Build history of the part. All positions in model axes, mm. A direction names the side the tool comes from. Give positions to 0.01 mm unless a question says otherwise; leave off trailing zeros. Write each loop counter-clockwise with the first axis right and the second up, starting at its lowest first coordinate (ties: lowest second). Pieces come first, ordered by that corner, then holes. Notation, with made-up numbers: (12, -27.75) -> (52, -27.75) arc R16 cw to (52, -10.75) -> close; hole circle Ø3 at (-32, 10). An arc over 180 degrees is marked (long way). Write item = value, one per line. Start each with the question number.
Q1. Wall check: line 1 (Y direction, x = 8.5, z = -23); line 2 (Z direction, x = 0, y = -187.5); line 3 (Y direction, x = 20.9, z = 0). Give the ranges that are in metal, low to high.
Q2. Drop flat-ended pins along their axis: P1, Ø1.5, axis at y = -106.5, z = 6.5, coming from the +X side; P2, Ø10, axis at x = -18.5, z = 10.5, coming from the +Y side; P3, Ø10, axis at y = -237, z = 8, coming from the -X side. Give the stop position or say it passes through.
Q3. Saw through at A-A, the plane y = -20. List the corners of the cut face in (x, z), then the cut area to 3 significant figures.
Q4. Tool access for faces 5 (the face through (-9.4, -351, 22.3)), 6 (the face through (-7.956, -414.86, -11.236)), 7 (the face through (22, -124, 0)), 8 (the face through (13.041, -414.86, 4.414)): list every direction of +Z, -Z, +X, -X, +Y, -Y with a clear straight run to the whole face (end or side of a thin tool).
Q5. Saw through at B-B, the plane y = -112. List the corners of the cut face in (x, z).
Q6. Mould opens along Y. For faces 1 (the face through (3, -425, -1)), 2 (the face through (4, -400, 0)), 3 (the face through (5.4, 1.1, 10)), 4 (the face through (23.846, -299.3, 7.509)) say: pulls with the +Y half, pulls with the -Y half, needs draft (parallel to the pull), parting line crosses it, or undercut.
from build123d import *

# Parameters (mm, degrees)
F0_R          = 25
F0_R_2        = 20
F1_DEPTH      = 400
F2_R          = 25
F3_DEPTH      = 5
F5_DEPTH      = 20
F7_D          = 5
F10_D         = 12
F10_DEPTH     = 6
F10_START     = 0.7306779
F10_TIP       = 3.6051637142
F12_DEPTH     = 2
F17_D         = 12
F17_DEPTH     = 6
F17_START     = 0.7306779
F17_TIP       = 3.6051637142
F19_D         = 12
F19_DEPTH     = 6
F19_START     = 0.7306779
F19_TIP       = 3.6051637142
F21_R         = 25
F21_R_2       = 24
F22_DEPTH     = 1
F24_R         = 25
F24_R_2       = 24
F25_DEPTH     = 1
F27_DEPTH     = 20
F28_T1_DEPTH  = 16.0381401647
F28_T3_DEPTH  = 31.2249898061
F28_T5_DEPTH  = 16.0381402184
F28_T7_DEPTH  = 16.0381401647
F28_T9_DEPTH  = 31.2249898061
F28_T11_DEPTH = 16.0381402184
F28_T13_DEPTH = 16.0381401647
F28_T15_DEPTH = 31.2249898061
F28_T17_DEPTH = 16.0381402184


# Not quite as in the source:
# - a fillet or chamfer that OpenCascade refuses, or shapes differently, is made with other operations: its cross-section is extruded or revolved along the edge and cut away or added


with BuildPart() as f1:
    # F0 (on Front) → F1 (new body)
    with BuildSketch(Plane.XZ):
        Circle(F0_R)
        Circle(F0_R_2, mode=Mode.SUBTRACT)
    extrude(amount=F1_DEPTH)

    # F2 (on face) → F3 (join)
    with BuildSketch(Plane.XZ.offset(400)):
        Circle(F2_R)
    extrude(amount=F3_DEPTH)

    # F4 (on face) → F5 (join)
    with BuildSketch(Plane.XZ.offset(405)):
        Polygon((-16.0628025015, -5.6190539991), (0.380358971, -17.013016167), (16.2978772735, -4.8955682433), (9.6922831285, 13.9873885984), (-10.3077168715, 13.540249811), align=None)
    extrude(amount=F5_DEPTH)

    # F7 (through all)
    with Locations(Plane.XZ.offset(425)):
        with Locations((0, 0)):
            Hole(F7_D / 2)

    # F10
    # its depths count from where the whole tool has entered the part; down to there all is cleared
    with Locations(Plane.YZ.offset(25).offset(-F10_START)):
        with Locations((-20, 0), (-130, 0)):
            Hole(F10_D / 2, depth=F10_DEPTH)
            with Locations((0, 0, -(F10_DEPTH + F10_TIP / 2))):  # 118° drill point
                Cone(0, F10_D / 2, F10_TIP, mode=Mode.SUBTRACT)

    # F11 (on face) → F12 (join)
    with BuildSketch(Plane(origin=(0, 0, 0), x_dir=(-1, 0, 0), z_dir=(0, 1, 0))):
        Polygon((12.5, -21.6506350946), (12.5, 21.6506350946), (-25, 0), align=None)
    extrude(amount=F12_DEPTH)

    # F17
    # its depths count from where the whole tool has entered the part; down to there all is cleared
    with Locations(Plane(origin=(-12.5, 0, -21.6506350946), x_dir=(0.8660254038, 0, -0.5), z_dir=(-0.5, 0, -0.8660254038)).offset(-F17_START)):
        with Locations((0, 20), (0, 130)):
            Hole(F17_D / 2, depth=F17_DEPTH)
            with Locations((0, 0, -(F17_DEPTH + F17_TIP / 2))):  # 118° drill point
                Cone(0, F17_D / 2, F17_TIP, mode=Mode.SUBTRACT)

    # F19
    # its depths count from where the whole tool has entered the part; down to there all is cleared
    with Locations(Plane(origin=(-12.5, 0, 21.6506350946), x_dir=(0.8660254038, 0, 0.5), z_dir=(-0.5, 0, 0.8660254038)).offset(-F19_START)):
        with Locations((0, -20), (0, -130)):
            Hole(F19_D / 2, depth=F19_DEPTH)
            with Locations((0, 0, -(F19_DEPTH + F19_TIP / 2))):  # 118° drill point
                Cone(0, F19_D / 2, F19_TIP, mode=Mode.SUBTRACT)

    # F21 (on offset) → F22 (cut)
    with BuildSketch(Plane.XZ.offset(250)):
        Circle(F21_R)
        Circle(F21_R_2, mode=Mode.SUBTRACT)
    extrude(amount=-F22_DEPTH, mode=Mode.SUBTRACT)

    # F24 (on offset) → F25 (cut)
    with BuildSketch(Plane.XZ.offset(350)):
        Circle(F24_R)
        Circle(F24_R_2, mode=Mode.SUBTRACT)
    extrude(amount=F25_DEPTH, mode=Mode.SUBTRACT)

    # F26 (on face) → F27 (cut)
    with BuildSketch(Plane(origin=(0, 2, 0), x_dir=(-1, 0, 0), z_dir=(0, 1, 0))):
        Polygon((-20, 0), (10, -17.3205080757), (10, 17.3205080757), align=None)
    extrude(amount=-F27_DEPTH, mode=Mode.SUBTRACT)

    # F28: fillet of radius 5 on 3 edges, made by hand

    # F28_s2 → F28_t1 (cut)
    with BuildSketch(Plane(origin=(27.4102540378, 0, 15.8253175473), x_dir=(0, 1, 0), z_dir=(-0.8660254038, 0, -0.5))):
        with BuildLine():
            ThreePointArc((0, 12.5), (1.472135955, 10.7360679775), (2, 8.5))
            Line((2, 8.5), (2, 12.5))
            Line((2, 12.5), (0, 12.5))
        make_face()
    extrude(amount=F28_T1_DEPTH, mode=Mode.SUBTRACT)

    # F28_s4 → F28_t3 (cut)
    with BuildSketch(Plane(origin=(13.5208172258, 0, 7.806247465), x_dir=(0, 1, 0), z_dir=(-0.8660254038, 0, -0.5))):
        with BuildLine():
            ThreePointArc((0, 12.5), (1.472135955, 10.7360679775), (2, 8.5))
            Line((2, 8.5), (2, 12.5))
            Line((2, 12.5), (0, 12.5))
        make_face()
    extrude(amount=F28_T3_DEPTH, mode=Mode.SUBTRACT)

    # F28_s6 → F28_t5 (cut)
    with BuildSketch(Plane(origin=(-13.5208171792, 0, -7.8062474381), x_dir=(0, 1, 0), z_dir=(-0.8660254038, 0, -0.5))):
        with BuildLine():
            ThreePointArc((0, 12.5), (1.472135955, 10.7360679775), (2, 8.5))
            Line((2, 8.5), (2, 12.5))
            Line((2, 12.5), (0, 12.5))
        make_face()
    extrude(amount=F28_T5_DEPTH, mode=Mode.SUBTRACT)

    # F28_s8 → F28_t7 (cut)
    with BuildSketch(Plane.XY.offset(-31.6506350946)):
        with BuildLine():
            ThreePointArc((-12.5, 0), (-10.7360679775, 1.472135955), (-8.5, 2))
            Line((-8.5, 2), (-12.5, 2))
            Line((-12.5, 2), (-12.5, 0))
        make_face()
    extrude(amount=F28_T7_DEPTH, mode=Mode.SUBTRACT)

    # F28_s10 → F28_t9 (cut)
    with BuildSketch(Plane.XY.offset(-15.61249493)):
        with BuildLine():
            ThreePointArc((-12.5, 0), (-10.7360679775, 1.472135955), (-8.5, 2))
            Line((-8.5, 2), (-12.5, 2))
            Line((-12.5, 2), (-12.5, 0))
        make_face()
    extrude(amount=F28_T9_DEPTH, mode=Mode.SUBTRACT)

    # F28_s12 → F28_t11 (cut)
    with BuildSketch(Plane.XY.offset(15.6124948762)):
        with BuildLine():
            ThreePointArc((-12.5, 0), (-10.7360679775, 1.472135955), (-8.5, 2))
            Line((-8.5, 2), (-12.5, 2))
            Line((-12.5, 2), (-12.5, 0))
        make_face()
    extrude(amount=F28_T11_DEPTH, mode=Mode.SUBTRACT)

    # F28_s14 → F28_t13 (cut)
    with BuildSketch(Plane(origin=(-27.4102540378, 0, 15.8253175473), x_dir=(0, 1, 0), z_dir=(0.8660254038, 0, -0.5))):
        with BuildLine():
            ThreePointArc((0, 12.5), (1.472135955, 10.7360679775), (2, 8.5))
            Line((2, 8.5), (2, 12.5))
            Line((2, 12.5), (0, 12.5))
        make_face()
    extrude(amount=F28_T13_DEPTH, mode=Mode.SUBTRACT)

    # F28_s16 → F28_t15 (cut)
    with BuildSketch(Plane(origin=(-13.5208172258, 0, 7.806247465), x_dir=(0, 1, 0), z_dir=(0.8660254038, 0, -0.5))):
        with BuildLine():
            ThreePointArc((0, 12.5), (1.472135955, 10.7360679775), (2, 8.5))
            Line((2, 8.5), (2, 12.5))
            Line((2, 12.5), (0, 12.5))
        make_face()
    extrude(amount=F28_T15_DEPTH, mode=Mode.SUBTRACT)

    # F28_s18 → F28_t17 (cut)
    with BuildSketch(Plane(origin=(13.5208171792, 0, -7.8062474381), x_dir=(0, 1, 0), z_dir=(0.8660254038, 0, -0.5))):
        with BuildLine():
            ThreePointArc((0, 12.5), (1.472135955, 10.7360679775), (2, 8.5))
            Line((2, 8.5), (2, 12.5))
            Line((2, 12.5), (0, 12.5))
        make_face()
    extrude(amount=F28_T17_DEPTH, mode=Mode.SUBTRACT)


solid = f1.part
Report:
q1.line_1 = -405 to -351, -350 to -250, -249 to 0
q1.line_2 = -25 to -20, 20 to 25
q1.line_3 = -405 to -136, -124 to -26, -14 to 1.6
q2.P1 = 24.33
q2.P2 = 0
q2.P3 = -24.82
q3.outline = (-17.33, -18.02) -> (-14.74, -13.52) arc R20 cw to (-14.74, 13.52) -> (-17.33, 18.02) arc R25 ccw to start; (-6.94, -24.02) arc R25 ccw to (24.27, -6) -> (19.08, -6) arc R20 cw to (-4.34, -19.52) -> close; (-6.94, 24.02) -> (-4.34, 19.52) arc R20 cw to (19.08, 6) -> (24.27, 6) arc R25 ccw to start
q3.area = 525 mm2
q4.face_5 = none
q4.face_6 = -Z, -X, -Y
q4.face_7 = +X
q4.face_8 = +Z, +X, -Y
q5.outline = circle Ø50 at (0, 0); hole circle Ø40 at (0, 0)
q6.face_1 = pulls with the -Y half
q6.face_2 = undercut
q6.face_3 = pulls with the +Y half
q6.face_4 = needs draft
